Design review of the part built by this model. Coordinates are the model's own, in mm. A direction names the side the tool comes from. Round coordinates to 2 decimals unless told otherwise and drop trailing zeros. Loops run counter-clockwise (first coordinate to the right, second up) from the corner with the lowest first, then second, coordinate; pieces in that order, holes last. Notation, with made-up numbers: M 83.25,-17.75 L 98.25,-17.75 A20 ccw 98.25,-4.75 Z; hole C 18,35 d9. An arc over 180 degrees is marked long. Use a Markdown table: item, result.
from build123d import *

# Parameters (mm, degrees)
SKETCH1_W           = 40
SKETCH1_H           = 3
SKETCH1_W_2         = 43
BOSS_EXTRUDE1_DEPTH = 10


with BuildPart() as part:
    # Sketch1 → Boss-Extrude1 (new body)
    with BuildSketch(Plane.XY):
        with Locations((0, 100)):
            Rectangle(SKETCH1_W, SKETCH1_H)
        with Locations((-81.5, 100)):
            Rectangle(SKETCH1_W_2, SKETCH1_H)
        with Locations((81.5, 100)):
            Rectangle(SKETCH1_W_2, SKETCH1_H)
        with Locations((81.5, -100)):
            Rectangle(SKETCH1_W_2, SKETCH1_H)
        with Locations((0, -100)):
            Rectangle(SKETCH1_W, SKETCH1_H)
        with Locations((-81.5, -100)):
            Rectangle(SKETCH1_W_2, SKETCH1_H)
        Polygon((88, -84.155339806), (103, -98.5), (103, -78.5), (100, -78.5), (100, -48.5), (103, -48.5), (103, -18.5), (100, -18.5), (100, 11.5), (103, 11.5), (103, 41.5), (100, 41.5), (100, 71.5), (103, 71.5), (103, 98.5), (60, 98.5), (20, 98.5), (-20, 98.5), (-60, 98.5), (-103, 98.5), (71.629441624, -68.5), (88, -68.5), align=None)
        Polygon((-103, -78.5), (-103, -98.5), (-60, -98.5), (-20, -98.5), (20, -98.5), (60, -98.5), (103, -98.5), (88, -84.155339806), (88, -85.5), (55, -85.5), (55, -68.5), (71.629441624, -68.5), (-103, 98.5), (-103, 71.5), (-100, 71.5), (-100, 41.5), (-103, 41.5), (-103, 11.5), (-100, 11.5), (-100, -18.5), (-103, -18.5), (-103, -48.5), (-100, -48.5), (-100, -78.5), align=None)
    extrude(amount=BOSS_EXTRUDE1_DEPTH)


solid = part.part
1. The part is to be moulded in two halves that separate along X. For faces 1 (the face through (81, -101.5, 5)), 2 (the face through (103, -34, 5)), 3 (the face through (72, -85.5, 5)), say which applies: pulls with the +X half, pulls with the -X half, needs draft (parallel to the pull), parting line crosses it, or undercut.
Check values:
| item | result |
|---|---|
| face 1 | needs draft |
| face 2 | pulls with the +X half |
| face 3 | undercut |
2. Machinability: for faces 4 (the face through (71, -68.5, 5)), 5 (the face through (-100, 57, 5)), 6 (the face through (-40, 98.5, 5)), 7 (the face through (40, -98.5, 5)), which of the approach directions +Z, -Z, +X, -X, +Y, -Y give a long, thin tool a straight path to every point of the face, cutting with its end or side? Answer none if there is none.
Check values:
| item | result |
|---|---|
| face 4 | +Z, -Z |
| face 5 | +Z, -Z, -X |
| face 6 | +Z, -Z, +Y |
| face 7 | +Z, -Z, -Y |
3. Wall thickness on line 1 along Y through (x, z) = (70.5, 3.75); line 2 along X through (y, z) = (-62.5, 2.25); line 3 along Y through (x, z) = (47, 5): over which ranges is each line inside the solid? List them lowest first. Write a range as from..to.
Check values:
| item | result |
|---|---|
| line 1 | y = -101.5..-85.5, -68.5..101.5 |
| line 2 | x = -100..100 |
| line 3 | y = -98.5..98.5 |
4. Take a section at C-C on x = -50. Give the boundary of the cut face in (y, z), and give its area (3 significant figures).
Check values:
| item | result |
|---|---|
| outline | M -98.5,0 L 98.5,0 L 98.5,10 L -98.5,10 Z |
| area | 1,970 mm² |
5. Insertion check: pin 1 (2 mm diameter, centred on x = -34.5, z = 8.5, fed in from -Y); pin 2 (3 mm diameter, centred on y = 63, z = 3.5, fed in from +X); pin 3 (3 mm diameter, centred on x = 30, y = -79, fed in from -Z); pin 4 (1 mm diameter, centred on x = 21.5, z = 5.5, fed in from +Y). Each pin has a flat end and moves straight along its axis. Give the tip position at first contact, or say it passes through.
Check values:
| item | result |
|---|---|
| pin 1 | stops at y = -98.5 |
| pin 2 | stops at x = 100 |
| pin 3 | stops at z = 0 |
| pin 4 | stops at y = 98.5 |
6. Take a section at B-B on y = -14. Give the boundary of the cut face in (x, z), and give its area (3 significant figures).
Check values:
| item | result |
|---|---|
| outline | M -100,0 L 100,0 L 100,10 L -100,10 Z |
| area | 2,000 mm² |
7. Take a section at A-A on x = 65. Give the boundary of the cut face in (y, z), and give its area (3 significant figures).
Check values:
| item | result |
|---|---|
| outline | M -101.5,0 L -85.5,0 L -85.5,10 L -101.5,10 Z; M -68.5,0 L 101.5,0 L 101.5,10 L -68.5,10 Z |
| area | 1,860 mm² |
